The listing builds one solid part. Answer for the finished solid, in the listing's coordinates (mm). Give positions to 0.01 mm unless a question says otherwise; leave off trailing zeros. Order: outer loops, then holes, each group sorted by start corner. A loop starts at its lowest first (then second) coordinate and runs counter-clockwise, first axis right, second up. Notation, with made-up numbers: (27, -37.75) - (43, -37.75) arc R17 ccw to (43, -22.75) - close; hole circle Ø11 at (80.25, 25.5). An arc over 180 degrees is marked (long way). Write each question's results on one line, items separated by ' | '. Start each with the question number.
1. Section A-A (y = 3.75) is taken. State how many separate pieces and enclosed holes the cut face has, and give its area (3 significant figures).
2. Determine the mould class of faces 1 (the face through (7, 8, 0)), 2 (the face through (9.55, 2.46, -8.46)), 3 (the face through (4.537, 8.619, -63.481)) for opening direction Z: released by +Z, released by -Z, zero draft, split by the parting line, or undercut.
3. Flat-ended cylindrical pins translate along their axes: pin 1 (5 mm diameter, centred on y = 10.5, z = -22.5, fed in from -X); pin 2 (4.5 mm diameter, centred on x = 8.5, z = -11, fed in from -Y). Find the tip coordinate at first contact, or state that the pin passes through.
4. Section C-C (x = 8.5) is taken. Give the vertices of the cut face in (y, z).
5. Section D-D (y = 10.25) is taken. Give the vertices of the cut face in (x, z).
6. Find the intervals of material crossed by L1, parallel to Z at x = 11, y = 2.25; L2, parallel to X at y = 3.5, z = -40.5; L3, parallel to Z at x = 6.5, y = 1, in increasing order.
7. Section B-B (z = -11) is taken. Give the vertices of the cut face in (x, y), and give its area (3 significant figures).
from build123d import *

# Parameters (mm, degrees)
SKETCH_1_W          = 13.5
SKETCH_1_H          = 68.4
EXTRUDE_1_DEPTH     = 17
SKETCH_2_R          = 2.75
CUT_EXTRUDE_1_DEPTH = 5
CUT_EXTRUDE_2_DEPTH = 17
EXTRUDE_2_DEPTH     = 5.5
FILLET_1_R          = 30
FILLET_2_R          = 1
SKETCH_8_W          = 4
SKETCH_8_H          = 19.960959335
CUT_EXTRUDE_5_DEPTH = 17


with BuildPart() as part:
    # ｽｹｯﾁ1 → ﾎﾞｽ - 押し出し1 (new body)
    with BuildSketch(Plane(origin=(0, 0, 0), x_dir=(1, 0, 0), z_dir=(0, 1, 0))):
        with Locations((6.75, 34.2)):
            Rectangle(SKETCH_1_W, SKETCH_1_H)
    extrude(amount=EXTRUDE_1_DEPTH)

    # ｽｹｯﾁ2 → ｶｯﾄ - 押し出し1 (cut)
    with BuildSketch(Plane.XZ):
        with Locations(Location((8.5, -47.4, 0), (0, 0, 270))):
            Circle(SKETCH_2_R)
        with Locations(Location((8.5, -11, 0), (0, 0, 90))):
            Circle(SKETCH_2_R)
    extrude(amount=-CUT_EXTRUDE_1_DEPTH, mode=Mode.SUBTRACT)

    # ｽｹｯﾁ3 → ｶｯﾄ - 押し出し2 (cut)
    with BuildSketch(Plane(origin=(0, 17, 0), x_dir=(1, 0, 0), z_dir=(0, 1, 0))):
        Polygon((6.75, 68.4), (0, 68.4), (0, 53.4), align=None)
    extrude(amount=-CUT_EXTRUDE_2_DEPTH, mode=Mode.SUBTRACT)

    # ｽｹｯﾁ4 → ﾎﾞｽ - 押し出し2 (add)
    with BuildSketch(Plane.XZ):
        Polygon((0, -47), (-4, -37), (-4, -27), (0, -27), align=None)
    extrude(amount=-EXTRUDE_2_DEPTH)

    # ﾌｨﾚｯﾄ1
    fillet_1_edges = [part.edges().sort_by_distance(p)[0] for p in [
        (0, 8.5, -53.4),
    ]]
    fillet(fillet_1_edges, radius=FILLET_1_R)

    # ﾌｨﾚｯﾄ2
    fillet_2_edges = [part.edges().sort_by_distance(p)[0] for p in [
        (6.75, 8.5, -68.4),
        (13.5, 8.5, -68.4),
        (13.5, 8.5, 0),
        (0, 8.5, 0),
    ]]
    fillet(fillet_2_edges, radius=FILLET_2_R)

    # ｽｹｯﾁ8 → ｶｯﾄ - 押し出し5 (cut)
    with BuildSketch(Plane(origin=(0, 17, 0), x_dir=(1, 0, 0), z_dir=(0, 1, 0))):
        with Locations((-2, 36.980479668)):
            Rectangle(SKETCH_8_W, SKETCH_8_H)
    extrude(amount=-CUT_EXTRUDE_5_DEPTH, mode=Mode.SUBTRACT)


solid = part.part
Reported:
1) separate pieces: 1 | enclosed holes: 2 | area: 822 mm²
2) face 1: released by +Z | face 2: undercut | face 3: released by -Z
3) pin 1: x = 0 | pin 2: y = 5
4) outline: (0, -68.4) - (17, -68.4) - (17, 0) - (0, 0) - (0, -8.25) - (5, -8.25) - (5, -13.75) - (0, -13.75) - (0, -44.65) - (5, -44.65) - (5, -50.15) - (0, -50.15) - close
5) outline: (0, -46.96) arc R30 ccw to (2.64, -59.27) - (6.48, -67.81) arc R1 ccw to (7.4, -68.4) - (12.5, -68.4) arc R1 ccw to (13.5, -67.4) - (13.5, -1) arc R1 ccw to (12.5, 0) - (1, 0) arc R1 ccw to (0, -1) - close
6) L1: -68.4 to -48.55, -46.25 to -12.15, -9.85 to 0 | L2: 0 to 13.5 | L3: -67.84 to -49.29, -45.51 to -12.89, -9.11 to 0
7) outline: (0, 0) - (5.75, 0) - (5.75, 5) - (11.25, 5) - (11.25, 0) - (13.5, 0) - (13.5, 17) - (0, 17) - close | area: 202 mm²
